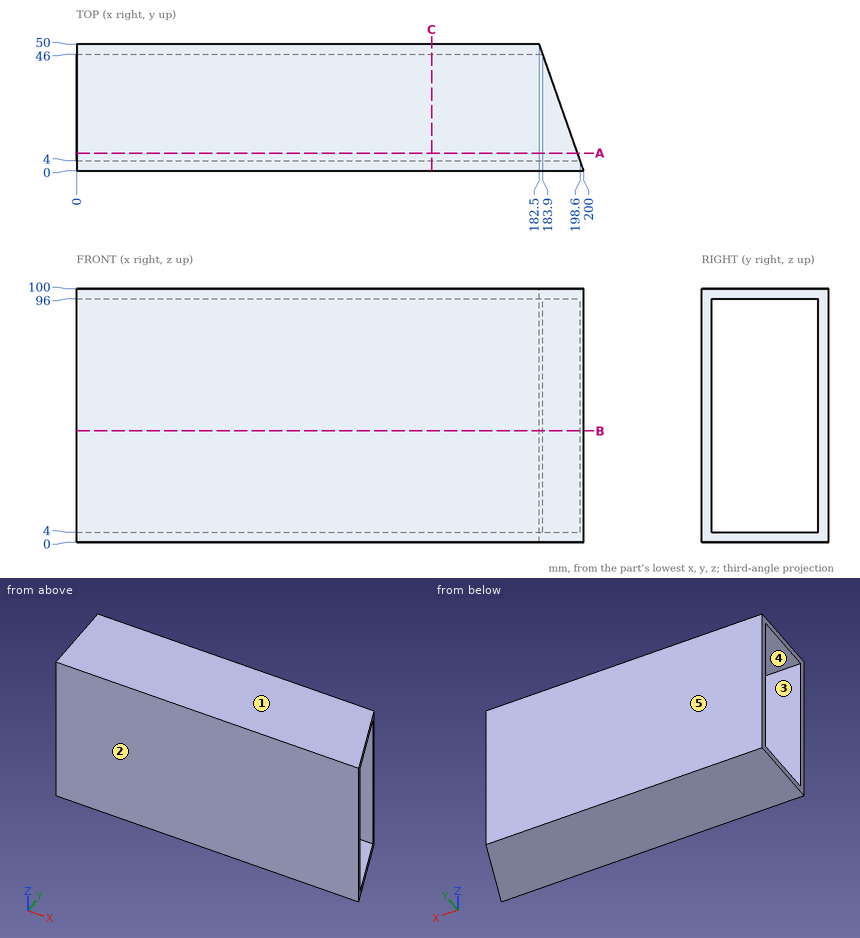
Study the drawing (mm; zero at the part's minimum x, y, z) and answer. A direction names the side the tool comes from. Round coordinates to 2 decimals unless told otherwise and drop trailing zeros. Order: outer loops, then holes, each group sorted by start corner. A loop starts at its lowest first (then second) coordinate and runs counter-clockwise, first axis right, second up. Notation, with made-up numbers: (-16.75, 19.5) - (19.25, 19.5) arc R35 ccw to (19.25, 56.5) - close; hole circle Ø3 at (55, -26.5). An arc over 180 degrees is marked (long way). Use one line per item in the form item = value. Start each with the question number.
(1) The part is cut by section B-B (z = 44). Give the vertices of the cut face in (x, y).
(2) The part is cut by section C-C (x = 140). Give the vertices of the cut face in (y, z).
(3) The part is cut by section A-A (y = 7). Give the vertices of the cut face in (x, z).
(4) Flat-ended cylindrical pins translate along their axes: pin 1 Ø10 at (x, z) = (26.5, 43) entering from -Y; pin 2 Ø6 at (y, z) = (45, 16) entering from +X. Find the tip coordinate at first contact, or state that the pin passes through.
(5) For the marked faces 4 and 5, determine the directions among +Z, -Z, +X, -X, +Y, -Y from which every point of the face is accessible in a straight line to the end or side of a thin tool.
(6) Determine the mould class of the marked faces 1, 2 and 3 for opening direction Y: +Y half, -Y half, draft (parallel to the pull), parting line (faces both ways), or undercut.
(7) Find the intervals of material crossed by line 1 along Z through (x, y) = (126.5, 25.5); line 2 along Y through (x, z) = (116.5, 56), in increasing order. Write a range as from..to.
Checked values:
q1.outline = (0, 0) - (200, 0) - (198.6, 4) - (0, 4) - close; (0, 46) - (183.9, 46) - (182.5, 50) - (0, 50) - close
q2.outline = (0, 0) - (50, 0) - (50, 100) - (0, 100) - close; hole (4, 4) - (46, 4) - (46, 96) - (4, 96) - close
q3.outline = (0, 0) - (197.55, 0) - (197.55, 4) - (0, 4) - close; (0, 96) - (197.55, 96) - (197.55, 100) - (0, 100) - close
q4.pin_1 = 0
q4.pin_2 = 183.9
q5.face_4 = +X, -X
q5.face_5 = +Z, -Z, +X, -X, +Y
q6.face_1 = draft
q6.face_2 = -Y half
q6.face_3 = undercut
q7.line_1 = 0..4, 96..100
q7.line_2 = 0..4, 46..50
